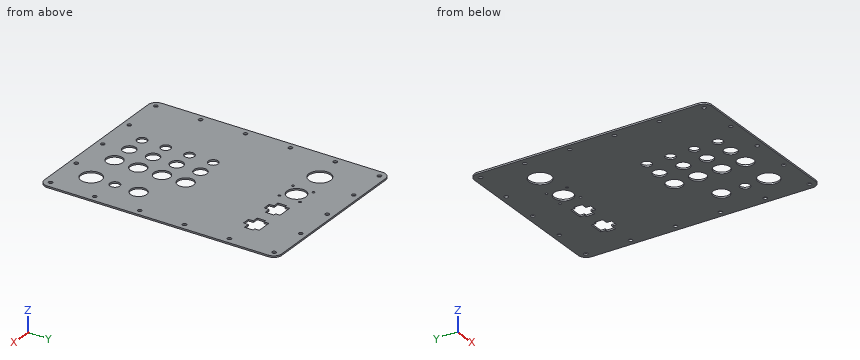
```python
from build123d import *

# Parameters (mm, degrees)
BOSS_EXTRUDE1_DEPTH = 2
SKETCH2_R           = 2.525
CUT_EXTRUDE1_DEPTH  = 187.021504133
SKETCH3_R           = 10.25
SKETCH3_R_2         = 8.25
SKETCH3_R_3         = 6.25
CUT_EXTRUDE2_DEPTH  = 187.021504133
CUT_EXTRUDE3_DEPTH  = 187.021504133
SKETCH6_R           = 12
SKETCH6_R_2         = 1.5
CUT_EXTRUDE4_DEPTH  = 187.021504133
CUT_EXTRUDE5_REACH  = 188.022
SKETCH7_R           = 13.75
CUT_EXTRUDE6_REACH  = 188.022
SKETCH8_R           = 13.05
SKETCH9_R           = 10.25
SKETCH9_R_2         = 6.25
CUT_EXTRUDE7_DEPTH  = 2


with BuildPart() as part:
    # Sketch1 → Boss-Extrude1 (new body)
    with BuildSketch(Plane.XY):
        with BuildLine():
            Line((-100, -150), (100, -150))
            ThreePointArc((100, -150), (107.071067812, -147.071067812), (110, -140))
            Line((110, -140), (110, 140))
            ThreePointArc((110, 140), (107.071067812, 147.071067812), (100, 150))
            Line((100, 150), (-100, 150))
            ThreePointArc((-100, 150), (-107.071067812, 147.071067812), (-110, 140))
            Line((-110, 140), (-110, -140))
            ThreePointArc((-110, -140), (-107.071067812, -147.071067812), (-100, -150))
        make_face()
    extrude(amount=BOSS_EXTRUDE1_DEPTH)

    # Sketch2 → Cut-Extrude1 (cut, through all)
    with BuildSketch(Plane.XY.offset(2)):
        with Locations((-101.414213562, 141.414213562)):
            Circle(SKETCH2_R)
        with Locations(Location((101.414213562, 141.414213562, 0), (0, 0, 180))):
            Circle(SKETCH2_R)
        with Locations((-51, 142)):
            Circle(SKETCH2_R)
        with Locations(Location((51, 142, 0), (0, 0, 180))):
            Circle(SKETCH2_R)
        with Locations((-102, 85.2)):
            Circle(SKETCH2_R)
        with Locations((-102, 28.4)):
            Circle(SKETCH2_R)
        with Locations(Location((102, 28.4, 0), (0, 0, 180))):
            Circle(SKETCH2_R)
        with Locations(Location((102, 85.2, 0), (0, 0, 180))):
            Circle(SKETCH2_R)
        with Locations((102, -28.4)):
            Circle(SKETCH2_R)
        with Locations((102, -85.2)):
            Circle(SKETCH2_R)
        with Locations((101.414213562, -141.414213562)):
            Circle(SKETCH2_R)
        with Locations((51, -142)):
            Circle(SKETCH2_R)
        with Locations(Location((-51, -142, 0), (0, 0, 180))):
            Circle(SKETCH2_R)
        with Locations(Location((-101.414213562, -141.414213562, 0), (0, 0, 180))):
            Circle(SKETCH2_R)
        with Locations(Location((-102, -85.2, 0), (0, 0, 180))):
            Circle(SKETCH2_R)
        with Locations(Location((-102, -28.4, 0), (0, 0, 180))):
            Circle(SKETCH2_R)
        with Locations((0, 142)):
            Circle(SKETCH2_R)
        with Locations(Location((0, -142, 0), (0, 0, 180))):
            Circle(SKETCH2_R)
    extrude(amount=-CUT_EXTRUDE1_DEPTH, mode=Mode.SUBTRACT)

    # Sketch3 → Cut-Extrude2 (cut, through all)
    with BuildSketch(Plane.XY.offset(2)):
        with Locations((23, -112)):
            Circle(SKETCH3_R)
        with Locations((-5.5, -112)):
            Circle(SKETCH3_R_2)
        with Locations((23, -82)):
            Circle(SKETCH3_R)
        with Locations((-5.5, -82)):
            Circle(SKETCH3_R_2)
        with Locations((23, -52)):
            Circle(SKETCH3_R)
        with Locations((-5.5, -52)):
            Circle(SKETCH3_R_2)
        with Locations((23, -22)):
            Circle(SKETCH3_R)
        with Locations((-5.5, -22)):
            Circle(SKETCH3_R_2)
        with Locations((-30, -112)):
            Circle(SKETCH3_R_3)
        with Locations((-30, -82)):
            Circle(SKETCH3_R_3)
        with Locations((-30, -52)):
            Circle(SKETCH3_R_3)
        with Locations((-30, -22)):
            Circle(SKETCH3_R_3)
    extrude(amount=-CUT_EXTRUDE2_DEPTH, mode=Mode.SUBTRACT)

    # Sketch5 → Cut-Extrude3 (cut, through all)
    with BuildSketch(Plane.XY.offset(2)):
        Polygon((10.875, 101.45), (10.875, 95.6), (7.75, 95.6), (7.75, 84.7), (15.175, 84.7), (15.175, 78.55), (24.825, 78.55), (24.825, 84.7), (32.25, 84.7), (32.25, 95.6), (29.125, 95.6), (29.125, 101.45), align=None)
        Polygon((50.875, 101.45), (50.875, 95.6), (47.75, 95.6), (47.75, 84.7), (55.175, 84.7), (55.175, 78.55), (64.825, 78.55), (64.825, 84.7), (72.25, 84.7), (72.25, 95.6), (69.125, 95.6), (69.125, 101.45), align=None)
    extrude(amount=-CUT_EXTRUDE3_DEPTH, mode=Mode.SUBTRACT)

    # Sketch6 → Cut-Extrude4 (cut, through all)
    with BuildSketch(Plane.XY.offset(2)):
        with Locations((-20, 90)):
            Circle(SKETCH6_R)
        with Locations((-7, 103)):
            Circle(SKETCH6_R_2)
        with Locations(Location((-33, 103, 0), (0, 0, 180))):
            Circle(SKETCH6_R_2)
        with Locations(Location((-7, 77, 0), (0, 0, 180))):
            Circle(SKETCH6_R_2)
        with Locations((-33, 77)):
            Circle(SKETCH6_R_2)
    extrude(amount=-CUT_EXTRUDE4_DEPTH, mode=Mode.SUBTRACT)

    # Sketch7 → Cut-Extrude5 (cut, up to next)
    with BuildSketch(Plane.XY.offset(2), mode=Mode.PRIVATE) as cut_extrude5_sk1:
        with Locations((-65, 90)):
            Circle(SKETCH7_R)
    cut_extrude5_tool1 = extrude(cut_extrude5_sk1.sketch, amount=-CUT_EXTRUDE5_REACH, mode=Mode.PRIVATE) & part.part
    add(cut_extrude5_tool1.solids().sort_by_distance((-65, 90, 2))[0], mode=Mode.SUBTRACT)

    # Sketch8 → Cut-Extrude6 (cut, up to next)
    with BuildSketch(Plane.XY.offset(2), mode=Mode.PRIVATE) as cut_extrude6_sk1:
        with Locations((68, -112)):
            Circle(SKETCH8_R)
    cut_extrude6_tool1 = extrude(cut_extrude6_sk1.sketch, amount=-CUT_EXTRUDE6_REACH, mode=Mode.PRIVATE) & part.part
    add(cut_extrude6_tool1.solids().sort_by_distance((68, -112, 2))[0], mode=Mode.SUBTRACT)

    # Sketch9 → Cut-Extrude7 (cut)
    with BuildSketch(Plane.XY.offset(2)):
        with Locations((68, -52)):
            Circle(SKETCH9_R)
        with Locations((68, -82)):
            Circle(SKETCH9_R_2)
    extrude(amount=-CUT_EXTRUDE7_DEPTH, mode=Mode.SUBTRACT)


solid = part.part
```
Verification items for the finished model (mm, model axes). Give positions to 0.01 mm unless a question says otherwise; leave off trailing zeros. Loops run counter-clockwise (first coordinate to the right, second up) from the corner with the lowest first, then second, coordinate; pieces in that order, holes last.
1. Section check B-B, the plane z = 1.1. Count the separate pieces of the cut face and the enclosed holes in it, then the cut area to 3 significant figures.
2. Thickness scan on line 1 (Y direction, x = 51, z = 1.5) (3 decimals); line 2 (Y direction, x = 23, z = 1.65); line 3 (Y direction, x = 68, z = 1.85). Record the ranges inside material, lowest first.
3. Go/stop test with a flat-tipped pin: pin 1 Ø15 at (x, y) = (-5.5, -52) entering from +Z. Record where the tip stops, or that it passes through.
4. Section check A-A, the plane x = -68. Enter the section's corners in (y, z), then the cut area to 3 significant figures.
Geometry says:
1. separate pieces: 1
1. enclosed holes: 41
1. area: 60,000 mm2
2. line 1: y = -150 to -144.525, -139.475 to 84.7, 101.45 to 139.475, 144.525 to 150
2. line 2: y = -150 to -122.25, -101.75 to -92.25, -71.75 to -62.25, -41.75 to -32.25, -11.75 to 78.55, 101.45 to 150
2. line 3: y = -150 to -125.05, -98.95 to -88.25, -75.75 to -62.25, -41.75 to 84.7, 101.45 to 150
3. pin 1: passes through
4. outline: (-150, 0) - (76.58, 0) - (76.58, 2) - (-150, 2) - close; (103.42, 0) - (150, 0) - (150, 2) - (103.42, 2) - close
4. area: 546 mm2
